For this review, use the dimensioned drawing (mm, ordinates from the lowest corner) and the shaded views. A direction names the side the tool comes from. Round coordinates to 2 decimals unless told otherwise and drop trailing zeros. Order: outer loops, then holes, each group sorted by start corner. A loop starts at its lowest first (then second) coordinate and runs counter-clockwise, first axis right, second up. Notation, with made-up numbers: (15.25, -6.5) - (40.25, -6.5) arc R10 cw to (40.25, 0.5) - close; hole circle Ø3 at (3, 86). An arc over 180 degrees is marked (long way). Write item = value, one per line.
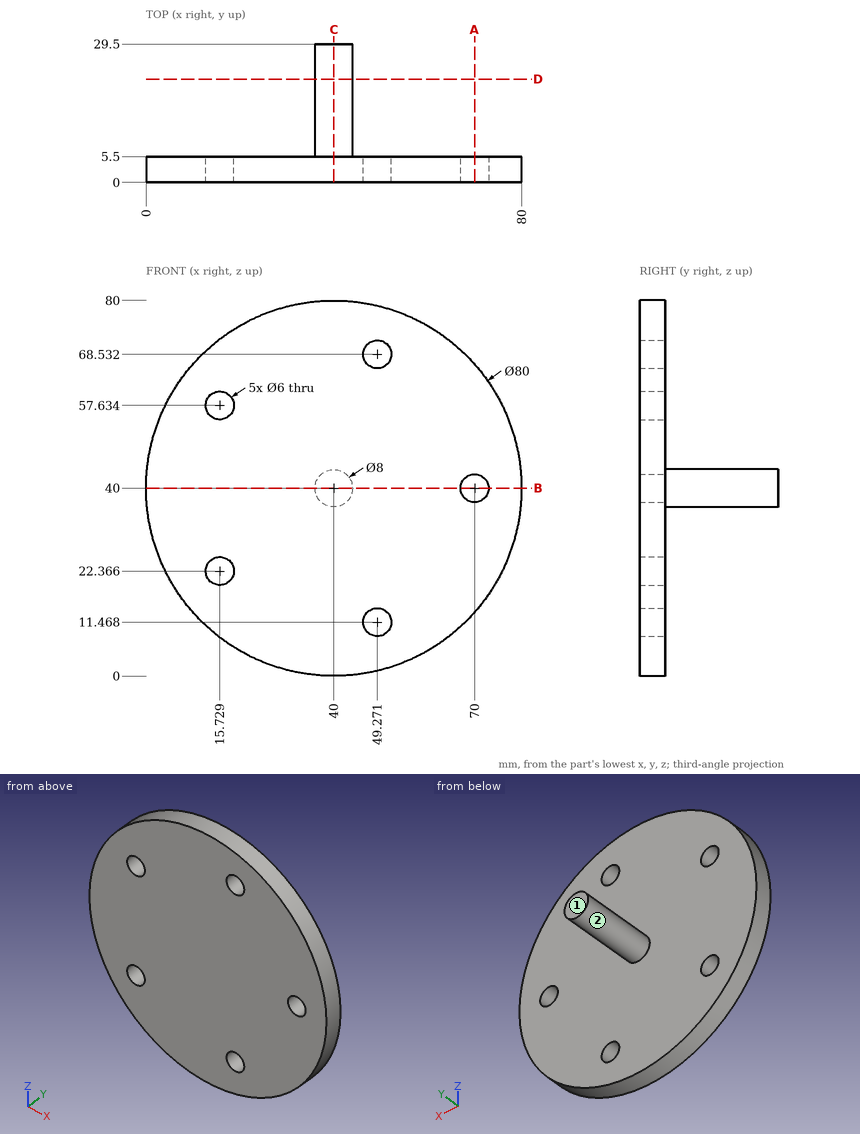
Item 1: For the marked faces 1 and 2, list the 3-axis set-ups (+Z, -Z, +X, -X, +Y, -Y) from which the entire face can be reached by the end or side of a thin tool; tool diameter is ignored.
Data:
face_1 = +Z, -Z, +X, -X, +Y
face_2 = +Y
Item 2: Insertion check: P1, Ø5, axis at x = 42, z = 32, coming from the -Y side; P2, Ø9.5, axis at x = 49.27, z = 68.53, coming from the +Y side; P3, Ø10, axis at y = 16, z = 40.5, coming from the -X side; P4, Ø4, axis at x = 69.5, y = 7, coming from the +Z side. Each pin has a flat end and moves straight along its axis. Give the tip position at first contact, or say it passes through.
Data:
P1 = 0
P2 = 5.5
P3 = 36
P4 = 68.39
Item 3: Take a section at D-D, the plane y = 22. State the section outline as (x, z) points.
Data:
outline = circle Ø8 at (40, 40)
Item 4: Take a section at C-C, the plane x = 40. State the section outline as (y, z) points.
Data:
outline = (0, 0) - (5.5, 0) - (5.5, 36) - (29.5, 36) - (29.5, 44) - (5.5, 44) - (5.5, 80) - (0, 80) - close
Item 5: Take a section at B-B, the plane z = 40. State the section outline as (x, y) points.
Data:
outline = (0, 0) - (67, 0) - (67, 5.5) - (44, 5.5) - (44, 29.5) - (36, 29.5) - (36, 5.5) - (0, 5.5) - close; (73, 0) - (80, 0) - (80, 5.5) - (73, 5.5) - close
Item 6: Take a section at A-A, the plane x = 70. State the section outline as (y, z) points.
Data:
outline = (0, 13.54) - (5.5, 13.54) - (5.5, 37) - (0, 37) - close; (0, 43) - (5.5, 43) - (5.5, 66.46) - (0, 66.46) - close
Item 7: For line 1 along Y through (x, z) = (31, 46); line 2 along X through (y, z) = (1.75, 69.5) (1 decimal); line 3 along X through (y, z) = (3.75, 9.5) (1 decimal), list the stretches that pass through material, from the lowest coordinate up. Write a range as [from, to].
Data:
line_1 = [0, 5.5]
line_2 = [13, 46.4], [52.1, 67]
line_3 = [14.1, 47], [51.5, 65.9]
